Input: part model. Units: mm. Frame: model coordinates. Face numbers are marked on the shaded views. Coordinates: 2 decimals unless noted, no trailing zeros. Write each loop counter-clockwise with the first axis right and the second up, starting at its lowest first coordinate (ties: lowest second). Pieces come first, ordered by that corner, then holes. Notation, with made-up numbers: (-21.75, 84.25) -> (14.25, 84.25) arc R12 cw to (14.25, 104.25) -> close; hole circle Ø1 at (-20, 33). An arc over 180 degrees is marked (long way). One line per question, with ' | ' between items. Start each with the question number.
```python
from build123d import *

# Parameters (mm, degrees)
AUFSATZ_LINEAR_AUSTRAGEN1_DEPTH = 849


with BuildPart() as part:
    # Skizze1 → Aufsatz-Linear austragen1 (new body)
    with BuildSketch(Plane(origin=(0, 0, 0), x_dir=(0, 0, -1), z_dir=(1, 0, 0))):
        with BuildLine():
            Line((49.569106164, 19.317466899), (477.280680476, 186))
            Line((477.280680476, 186), (539.372310058, 26.671316029))
            Line((539.372310058, 26.671316029), (470.933041974, 0))
            Line((470.933041974, 0), (413.328001817, 0))
            ThreePointArc((413.328001817, 0), (402.093085354, 9.319853414), (409.17705944, 22.083094646))
            Line((409.17705944, 22.083094646), (474.376050862, 47.491649613))
            ThreePointArc((474.376050862, 47.491649613), (479.900973413, 52.788240457), (480.062428312, 60.440205962))
            Line((480.062428312, 60.440205962), (455.371020057, 123.798980874))
            ThreePointArc((455.371020057, 123.798980874), (450.074429213, 129.323903425), (442.422463709, 129.485358324))
            Line((442.422463709, 129.485358324), (110.1597759, 0))
            Line((110.1597759, 0), (53.200195614, 0))
            ThreePointArc((53.200195614, 0), (43.372310058, 8.152659884), (49.569106164, 19.317466899))
        make_face()
    extrude(amount=AUFSATZ_LINEAR_AUSTRAGEN1_DEPTH)


solid = part.part
```
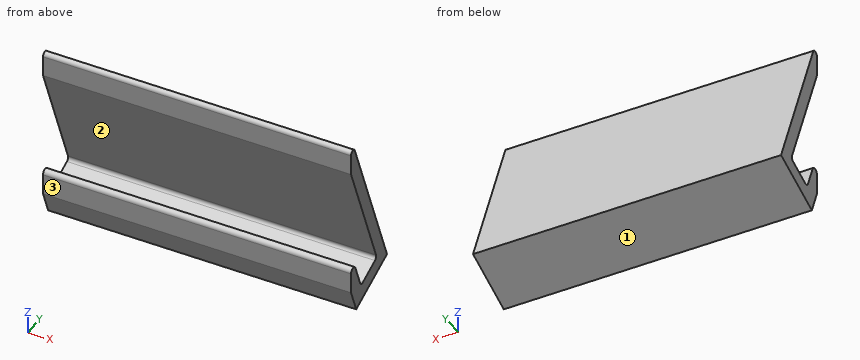
1) First-contact query: P1, Ø8, axis at x = 263, z = -309.5, coming from the -Y side; P2, Ø1.5, axis at x = 122, y = 118.5, coming from the -Z side; P3, Ø8, axis at x = 679, z = -111.5, coming from the +Y side. Flat tips, straight axial feed; report the tip coordinate or a pass-through.
2) Section B-B, the plane x = 401.5. Return loops of the section in (y, z), then the cut area to 3 significant figures.
3) Section C-C, the plane z = -341. Return loops of the section in (x, y), then the cut area to 3 significant figures.
4) Section D-D, the plane y = 161.5. Return loops of the section in (x, z).
5) Section A-A, the plane y = 83.5. Return loops of the section in (x, z), then the cut area to 3 significant figures.
6) Ray query, line 1 (Y direction, x = 462.5, z = -452); line 2 (Y direction, x = 382.5, z = -446); line 3 (Y direction, x = 66, z = -276). Return the intervals inside material, ascending.
7) Pull-direction query (Z, two-part tool) for the marked faces 1, 2 and 3; classes: released by +Z, released by -Z, zero draft, split by the parting line, or undercut.
Answer block:
1) P1: stops at y = 76.13 | P2: stops at z = -503.88 | P3: stops at y = 45.01
2) outline: (0, -470.93) -> (26.67, -539.37) -> (186, -477.28) -> (19.32, -49.57) arc R10 ccw to (0, -53.2) -> (0, -110.16) -> (129.49, -442.42) arc R10 cw to (123.8, -455.37) -> (60.44, -480.06) arc R10 cw to (47.49, -474.38) -> (22.08, -409.18) arc R11.43 ccw to (0, -413.33) -> close | area: 26,900 mm2
3) outline: (0, 89.96) -> (849, 89.96) -> (849, 132.89) -> (0, 132.89) -> close | area: 36,400 mm2
4) outline: (0, -486.83) -> (849, -486.83) -> (849, -414.41) -> (0, -414.41) -> close
5) outline: (0, -517.23) -> (849, -517.23) -> (849, -471.08) -> (0, -471.08) -> close; (0, -324.42) -> (849, -324.42) -> (849, -214.26) -> (0, -214.26) -> close | area: 133,000 mm2
6) line 1: y = 0 to 38.77, 128.21 to 176.15 | line 2: y = 0 to 36.43, 130.17 to 173.81 | line 3: y = 64.63 to 107.56
7) face 1: released by -Z | face 2: undercut | face 3: zero draft
